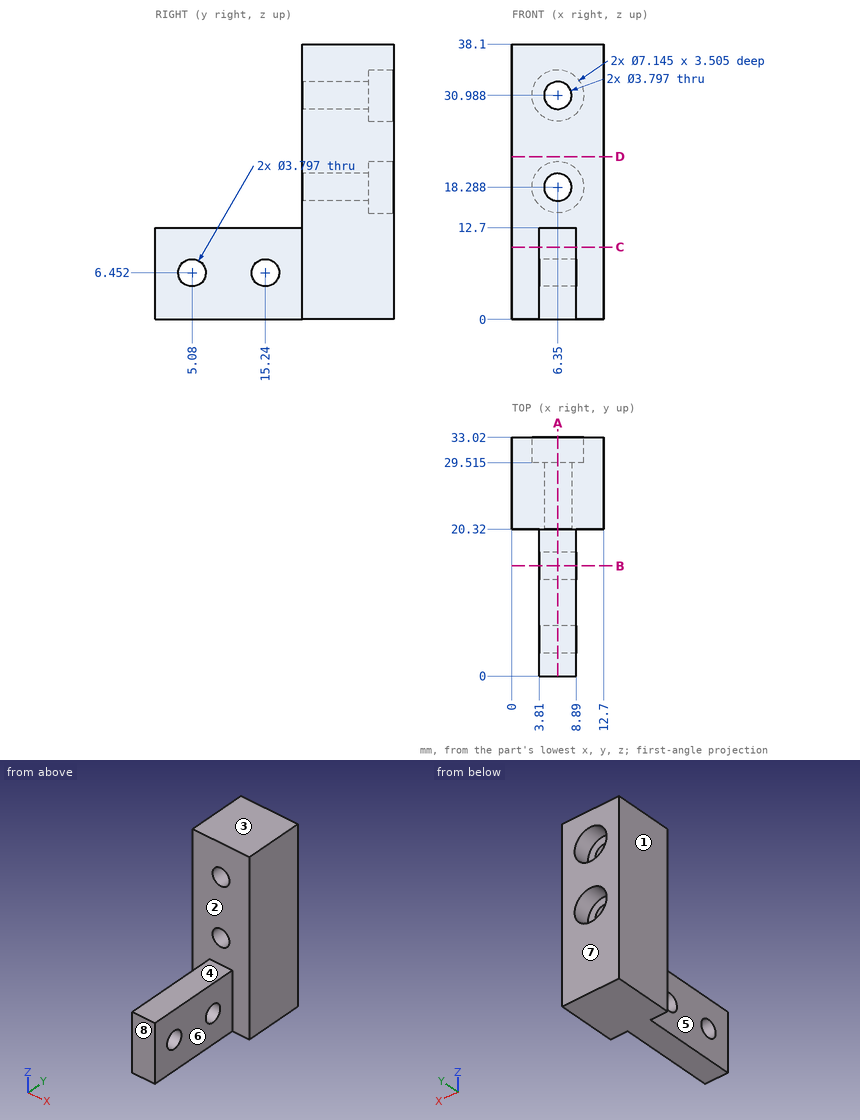
Geometry: see drawing. Coordinates: mm, zero at the bounding-box minimum. A direction names the side the tool comes from. Give positions to 0.01 mm unless a question says otherwise; leave off trailing zeros. Write each loop counter-clockwise with the first axis right and the second up, starting at its lowest first coordinate (ties: lowest second). Pieces come first, ordered by that corner, then holes. Notation, with made-up numbers: M 29.25,32 L 42.25,32 A16 ccw 42.25,60 Z; hole C 34.5,63 d11. An arc over 180 degrees is marked long. Return JSON: item names as keys, results as strings. Group by question number.
1) Cut plane C-C, the plane z = 10. Output: boundary loops of the cut face in (x, y).
2) Ray query, L1, parallel to Z at x = 6.35, y = 30.7 (1 decimal); L2, parallel to Y at x = 8, z = 7.5; L3, parallel to Y at x = 10.25, z = 24.5. Return the intervals inside material, ascending.
3) Cut plane A-A, the plane x = 6.35. Output: boundary loops of the cut face in (y, z) (1 decimal), then the cut area to 3 significant figures.
4) Cut plane B-B, the plane y = 15.24. Output: boundary loops of the cut face in (x, z), then the cut area to 3 significant figures.
5) Set-up query: the marked faces 1, 2, 3, 4 and 5. Return all of +Z, -Z, +X, -X, +Y, -Y with unobstructed straight access to the full face (end or side cutting, diameter ignored); none if empty.
6) Cut plane D-D, the plane z = 22.5. Output: boundary loops of the cut face in (x, y), then the cut area to 3 significant figures.
7) Draft query along Y for the marked faces 6, 7 and 8. Return one class per face: released by +Y, released by -Y, zero draft, split by the parting line, or undercut.
8) First-contact query: pin 1 Ø6 at (x, z) = (6.35, 30.988) entering from +Y (1 decimal); pin 2 Ø6 at (x, z) = (6.35, 18.288) entering from -Y; pin 3 Ø2 at (y, z) = (15.5, 5.5) entering from +X; pin 4 Ø3.5 at (y, z) = (5.08, 6.45) entering from +X. Flat tips, straight axial feed; report the tip coordinate or a pass-through.
Data:
{
 "1": {"outline": "M 0,20.32 L 3.81,20.32 L 3.81,0 L 8.89,0 L 8.89,20.32 L 12.7,20.32 L 12.7,33.02 L 0,33.02 Z"},
 "2": {"L1": "z = 0 to 14.7, 21.9 to 27.4, 34.6 to 38.1", "L2": "y = 0 to 3.5, 6.66 to 13.66, 16.82 to 33.02", "L3": "y = 20.32 to 33.02"},
 "3": {"outline": "M 0,0 L 33,0 L 33,14.7 L 29.5,14.7 L 29.5,16.4 L 20.3,16.4 L 20.3,12.7 L 0,12.7 Z; M 20.3,20.2 L 29.5,20.2 L 29.5,21.9 L 33,21.9 L 33,27.4 L 29.5,27.4 L 29.5,29.1 L 20.3,29.1 Z; M 20.3,32.9 L 29.5,32.9 L 29.5,34.6 L 33,34.6 L 33,38.1 L 20.3,38.1 Z; hole C 5.1,6.5 d3.8; hole C 15.2,6.5 d3.8", "area": "599 mm²"},
 "4": {"outline": "M 3.81,0 L 8.89,0 L 8.89,4.55 L 3.81,4.55 Z; M 3.81,8.35 L 8.89,8.35 L 8.89,12.7 L 3.81,12.7 Z", "area": "45.2 mm²"},
 "5": {"face 1": "+Z, -Z, -X, +Y, -Y", "face 2": "+Z, -Y", "face 3": "+Z, +X, -X, +Y, -Y", "face 4": "+Z, +X, -X, -Y", "face 5": "+Z, -Z, -X, -Y"},
 "6": {"outline": "M 0,20.32 L 12.7,20.32 L 12.7,33.02 L 0,33.02 Z", "area": "161 mm²"},
 "7": {"face 6": "zero draft", "face 7": "released by +Y", "face 8": "released by -Y"},
 "8": {"pin 1": "stops at y = 29.5", "pin 2": "stops at y = 20.32", "pin 3": "stops at x = 8.89", "pin 4": "passes through"}
}
